from build123d import *

# Parameters (mm, degrees)
F0_W     = 102.955818
F0_H     = 91.223456
F1_DEPTH = 25.4
F2_W     = 91.223456
F2_H     = 3.111502
F3_DEPTH = 101.6
F4_W     = 91.223456
F4_H     = 3.175
F5_DEPTH = 101.6
F6_W     = 102.955818
F6_H     = 3.175
F7_DEPTH = 88.9


with BuildPart() as f1:
    # F0 (on Top) → F1 (new body)
    with BuildSketch(Plane.XY):
        Rectangle(F0_W, F0_H)
    extrude(amount=F1_DEPTH)

    # F2 (on face) → F3 (cut)
    with BuildSketch(Plane(origin=(-51.477909, 0, 0), x_dir=(0, -1, 0), z_dir=(-1, 0, 0))):
        with Locations((0, 21.836062)):
            Rectangle(F2_W, F2_H)
    extrude(amount=-F3_DEPTH, mode=Mode.SUBTRACT)

    # F4 (on face) → F5 (cut)
    with BuildSketch(Plane.YZ.offset(51.477909)):
        with Locations((0, 13.6525)):
            Rectangle(F4_W, F4_H)
    extrude(amount=-F5_DEPTH, mode=Mode.SUBTRACT)

    # F6 (on face) → F7 (cut)
    with BuildSketch(Plane.XZ.offset(45.611728)):
        with Locations((0, 4.532312)):
            Rectangle(F6_W, F6_H)
    extrude(amount=-F7_DEPTH, mode=Mode.SUBTRACT)


solid = f1.part
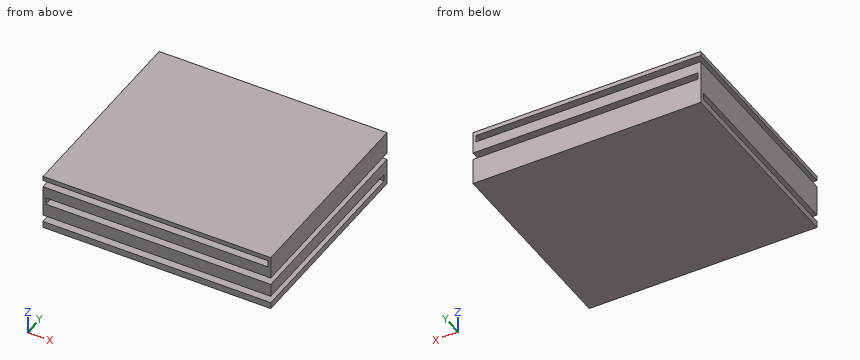
Build history of the part. All positions in model axes, mm. Coordinates: 2 decimals unless noted, no trailing zeros. Write each loop counter-clockwise with the first axis right and the second up, starting at its lowest first coordinate (ties: lowest second). Pieces come first, ordered by that corner, then holes.
(1) Drill centre lines: line 1 (Z direction, x = -25, y = 39.5) (3 decimals); line 2 (Y direction, x = -14, z = 5); line 3 (X direction, y = 18, z = 23.25). Where is each one in solid material? Low to high.
(2) Cut at C-C on z = 21.5. List the corners of the cut face in (x, y), and give its area (3 significant figures).
(3) Pin check, flat tip, straight feed: pin 1 Ø1 at (x, z) = (18.5, 21.5) entering from -Y. Stop position of the tip, or through.
(4) Cut at A-A on x = 40. List the corners of the cut face in (y, z) (3 decimals), and give its area (3 significant figures).
(5) Cut at B-B on y = 37.5. List the corners of the cut face in (x, z) (3 decimals), and give its area (3 significant figures).
Working result:
1. line 1: z = 0 to 2.945, 6.12 to 12.065, 15.24 to 20.28, 23.392 to 25.4
1. line 2: y = 43.29 to 45.61
1. line 3: x = 50.12 to 51.48
2. outline: (50.12, -45.61) - (51.48, -45.61) - (51.48, 45.61) - (50.12, 45.61) - close
2. area: 124 mm2
3. pin 1: passes through
4. outline: (-45.612, 0) - (45.612, 0) - (45.612, 12.065) - (-45.612, 12.065) - (-45.612, 6.12) - (43.288, 6.12) - (43.288, 2.945) - (-45.612, 2.945) - close; (-45.612, 15.24) - (45.612, 15.24) - (45.612, 20.28) - (-45.612, 20.28) - close; (-45.612, 23.392) - (45.612, 23.392) - (45.612, 25.4) - (-45.612, 25.4) - close
4. area: 1,460 mm2
5. outline: (-51.478, 0) - (51.478, 0) - (51.478, 2.945) - (-51.478, 2.945) - close; (-51.478, 6.12) - (51.478, 6.12) - (51.478, 12.065) - (-50.122, 12.065) - (-50.122, 15.24) - (51.478, 15.24) - (51.478, 25.4) - (-51.478, 25.4) - (-51.478, 23.392) - (50.122, 23.392) - (50.122, 20.28) - (-51.478, 20.28) - close
5. area: 1,650 mm2
